```python
from build123d import *

# Parameters (mm, degrees)
F1_DEPTH = 3.175
F2_R     = 5.08


# Not quite as in the source:
# - a length typed as a fraction of an inch, garbled in the dataset ("3 / 203.2 mm" for 3/8 in), is restored


with BuildPart() as f1:
    # F0 (on Top) → F1 (new body)
    with BuildSketch(Plane.XY):
        with BuildLine():
            Line((0, 6.35), (0, 0))
            Line((0, 0), (39.228014, 0))
            Line((39.228014, 0), (39.228014, -3.175))
            Line((39.228014, -3.175), (0, -3.175))
            Line((0, -3.175), (0, -30.5298216847))
            Line((0, -30.5298216847), (0, -127.8741553825))
            ThreePointArc((0, -127.8741553825), (11.1624656807, -154.8181574015), (38.1091467085, -165.9741542846))
            Line((38.1091467085, -165.9741542846), (51.0104592901, -165.9710570523))
            ThreePointArc((51.0104592901, -165.9710570523), (54.1114045686, -163.4743163552), (52.3355938941, -159.9111615484))
            ThreePointArc((52.3355938941, -159.9111615484), (40.2763953072, -152.7327194477), (30, -143.175))
            ThreePointArc((30, -143.175), (22.0311793243, -104.8602527123), (45, -73.175))
            ThreePointArc((45, -73.175), (58.4492609505, -39.4498416322), (60, -3.175))
            Line((60, -3.175), (60, 0))
            Line((60, 0), (60, 6.35))
            Line((60, 6.35), (39.228014, 6.35))
            Line((39.228014, 6.35), (0, 6.35))
        make_face()
    extrude(amount=F1_DEPTH)

    # F2
    f2_edges = [f1.edges().sort_by_distance(p)[0] for p in [
        (60, 6.35, 1.5875),
        (0, 6.35, 1.5875),
        (45, -73.175, 1.5875),
    ]]
    fillet(f2_edges, radius=F2_R)


solid = f1.part
```
Geometry: final body of the model. Coordinates: model frame, mm. A direction names the side the tool comes from. Round coordinates to 2 decimals unless told otherwise and drop trailing zeros. Write each loop counter-clockwise with the first axis right and the second up, starting at its lowest first coordinate (ties: lowest second). Pieces come first, ordered by that corner, then holes.
Item 1: Mould query, pull axis Y, two halves, no side actions, for faces 6 (the face through (0, -65, 2)), 7 (the face through (1.449, 4.822, 1.61)), 8 (the face through (39.228, -2, 2)), 9 (the face through (10.87, -154.52, 1.57)). Classes: +Y half, -Y half, draft (parallel to the pull), parting line (faces both ways), or undercut.
Item 2: Section query A-A (x = 42.5). Return loops of the section in (y, z) (3 decimals).
Item 3: Material intervals for L1, parallel to Y at x = 15.5, z = 1.55 (3 decimals); L2, parallel to Y at x = 38, z = 2.65 (3 decimals); L3, parallel to Y at x = 6.5, z = 3 (3 decimals), sorted ascending.
Item 4: Section query B-B (x = 33). Return loops of the section in (y, z) (3 decimals).
Item 5: Section query D-D (y = -84.5). Return loops of the section in (x, z) (3 decimals), plus the area to 3 significant figures.
Item 6: Section query C-C (y = -64.5). Return loops of the section in (x, z) (3 decimals), plus the area to 3 significant figures.
Item 7: Pin query (flat end, axial travel): P1, Ø1.5, axis at x = 25.5, y = -133, coming from the -Z side; P2, Ø1.6, axis at y = -0.5, z = 1, coming from the +X side; P3, Ø8, axis at x = 34, y = -28, coming from the -Z side; P4, Ø1, axis at y = -2, z = 1, coming from the -X side. Return the tip coordinate at first contact, or that it passes through.
Item 8: Set-up query: faces 1 (the face through (60, -1, 2)), 2 (the face through (20, -3.175, 2)), 3 (the face through (23, -79, 3.175)), 4 (the face through (40.434, -152.851, 1.565)), 5 (the face through (30, 6.35, 2)). Return all of +Z, -Z, +X, -X, +Y, -Y with unobstructed straight access to the full face (end or side cutting, diameter ignored); none if empty.
Completed:
1. face 6: draft
1. face 7: +Y half
1. face 8: undercut
1. face 9: -Y half
2. outline: (-165.973, 0) - (-154.328, 0) - (-154.328, 3.175) - (-165.973, 3.175) - close; (-74.735, 0) - (6.35, 0) - (6.35, 3.175) - (-74.735, 3.175) - close
3. L1: y = -158.547 to -3.175, 0 to 6.35
3. L2: y = -165.974 to -150.948, -78.131 to -3.175, 0 to 6.35
3. L3: y = -149.159 to -3.175, 0 to 6.35
4. outline: (-165.631, 0) - (-146.403, 0) - (-146.403, 3.175) - (-165.631, 3.175) - close; (-83.052, 0) - (-3.175, 0) - (-3.175, 3.175) - (-83.052, 3.175) - close; (0, 0) - (6.35, 0) - (6.35, 3.175) - (0, 3.175) - close
5. outline: (0, 0) - (31.777, 0) - (31.777, 3.175) - (0, 3.175) - close
5. area: 101 mm2
6. outline: (0, 0) - (49.763, 0) - (49.763, 3.175) - (0, 3.175) - close
6. area: 158 mm2
7. P1: passes through
7. P2: stops at x = 60
7. P3: stops at z = 0
7. P4: stops at x = 39.23
8. face 1: +Z, -Z, +X, +Y
8. face 2: +Z, -Z, -X
8. face 3: +Z, +X, -X, +Y, -Y
8. face 4: +Z, -Z, +X
8. face 5: +Z, -Z, +X, -X, +Y
